Build history of the part. All positions in model axes, mm. A direction names the side the tool comes from. Give positions to 0.01 mm unless a question says otherwise; leave off trailing zeros. Loops run counter-clockwise (first coordinate to the right, second up) from the corner with the lowest first, then second, coordinate; pieces in that order, holes last. Notation, with made-up numbers: M 65,28.25 L 102,28.25 A14 cw 102,44.25 Z; hole C 16,-34 d7. An arc over 180 degrees is marked long. Put each result on its own line as item: value.
```python
from build123d import *

# Parameters (mm, degrees)
F1_DEPTH = 970
F2_W     = 35
F2_H     = 30
F3_DEPTH = 2.3
F4_W     = 2.4
F4_H     = 1
F5_DEPTH = 30.001


with BuildPart() as f1:
    # F0 (on Right) → F1 (new body)
    with BuildSketch(Plane.YZ):
        Polygon((0, 20), (0, 0), (2.3, 0), (2.3, 17.7), (27.7, 17.7), (27.7, 0), (30, 0), (30, 20), align=None)
    extrude(amount=F1_DEPTH)

    # F2 (on face) → F3 (cut)
    with BuildSketch(Plane.XY.offset(20)):
        with Locations((17.5, 15)):
            Rectangle(F2_W, F2_H)
        with Locations((952.5, 15)):
            Rectangle(F2_W, F2_H)
    extrude(amount=-F3_DEPTH, mode=Mode.SUBTRACT)

    # F4 (on face) → F5 (cut, through all)
    with BuildSketch(Plane.XZ):
        with Locations((33.8, 0.5)):
            Rectangle(F4_W, F4_H)
        with Locations((6.2, 0.5)):
            Rectangle(F4_W, F4_H)
        with Locations((936.2, 0.5)):
            Rectangle(F4_W, F4_H)
        with Locations((963.8, 0.5)):
            Rectangle(F4_W, F4_H)
    extrude(amount=-F5_DEPTH, mode=Mode.SUBTRACT)


solid = f1.part
```
Q1. Slice it at C-C (y = 13). List the corners of the cut face in (x, z), and give its area (3 significant figures).
Here are the results:
outline: M 35,17.7 L 935,17.7 L 935,20 L 35,20 Z
area: 2,070 mm²
Q2. Probe line 1 (Y direction, x = 75, z = 17); line 2 (Z direction, x = 267.5, y = 3.75); line 3 (X direction, y = 11.5, z = 18). List the from-to ranges inside material, lowest first. Write a range as from..to.
Here are the results:
line 1: 0..2.3, 27.7..30
line 2: 17.7..20
line 3: 35..935
Q3. Slice it at A-A (z = 5.25). List the corners of the cut face in (x, y), and give its area (3 significant figures).
Here are the results:
outline: M 0,0 L 970,0 L 970,2.3 L 0,2.3 Z; M 0,27.7 L 970,27.7 L 970,30 L 0,30 Z
area: 4,460 mm²
Q4. Drop flat-ended pins along their axis: pin 1 Ø2 at (x, y) = (618, 7) entering from -Z; pin 2 Ø2.5 at (x, y) = (24.5, 29.5) entering from +Z; pin 3 Ø0.7 at (x, y) = (6.5, 29) entering from -Z. Give the stop position or say it passes through.
Here are the results:
pin 1: z = 17.7
pin 2: z = 17.7
pin 3: z = 1
Q5. Tool access for faces 4 (the flat face through (479, 15, 17.7)), 5 (the flat face through (479, 15, 20)): list every direction of +Z, -Z, +X, -X, +Y, -Y with a clear straight run to the whole face (end or side of a thin tool).
Here are the results:
face 4: -Z, +X, -X
face 5: +Z, +X, -X, +Y, -Y
Q6. Slice it at B-B (x = 492.5). List the corners of the cut face in (y, z).
Here are the results:
outline: M 0,0 L 2.3,0 L 2.3,17.7 L 27.7,17.7 L 27.7,0 L 30,0 L 30,20 L 0,20 Z
Q7. Mould opens along Y. For faces 1 (the flat face through (478, 2.3, 9)), 2 (the flat face through (478, 0, 10)), 3 (the flat face through (478, 30, 10)) say: pulls with the +Y half, pulls with the -Y half, needs draft (parallel to the pull), parting line crosses it, or undercut.
Here are the results:
face 1: undercut
face 2: pulls with the -Y half
face 3: pulls with the +Y half
